Build history of the part. All positions in model axes, mm. A direction names the side the tool comes from. Give positions to 0.01 mm unless a question says otherwise; leave off trailing zeros. Loops run counter-clockwise (first coordinate to the right, second up) from the corner with the lowest first, then second, coordinate; pieces in that order, holes last. Notation, with made-up numbers: (47, 47) - (69, 47) arc R37 cw to (69, 85) - close; hole circle Ø2 at (42.5, 74.25). An arc over 180 degrees is marked (long way). Return JSON: item names as keys, results as strings. Group by question number.
1) Slice it at B-B (x = -29.4). List the corners of the cut face in (y, z).
2) Drill centre lines: probe 1 along Y at (x, z) = (-38.4, 1.1); probe 2 along Y at (x, z) = (-29.4, 1.3); probe 3 along Y at (x, z) = (-27.5, 4.05). Where is each one in solid material? Low to high. Write a range as from..to.
3) Drop flat-ended pins along their axis: pin 1 (0.6 mm diameter, centred on x = -28.5, z = 3, fed in from -Y); pin 2 (1.8 mm diameter, centred on x = -38.4, y = -23, fed in from -Z); pin 3 (1.6 mm diameter, centred on y = -2, z = 3.5, fed in from -X); pin 4 (2.5 mm diameter, centred on x = -29.4, y = 1.2, fed in from +Z). Give the stop position or say it passes through.
4) Mould opens along X. For faces 1 (the face through (-39.55, -0.35, 1.28)), 2 (the face through (-29, -3.6, 4)), 3 (the face through (-40.5, -14, 1)) say: released by +X, released by -X, zero draft, split by the parting line, or undercut.
5) Slice it at D-D (x = -38.4). List the corners of the cut face in (y, z).
6) Slice it at A-A (y = -30.2). List the corners of the cut face in (x, z).
7) 3-axis set-ups, long thin cutter, end or side, ignore diameter. For faces 4 (the face through (-30, -4, 1)), 5 (the face through (-29, -27.8, 4)), 6 (the face through (-32, -2, 4)), 7 (the face through (-29, -25, 4)), 8 (the face through (-26.3, -26, 4)): which of +Z, -Z, +X, -X, +Y, -Y reach the whole face in a straight line?
8) Slice it at C-C (z = 3.15). List the corners of the cut face in (x, y).
```python
from build123d import *

# Parameters (mm, degrees)
TYPE_C_PROFILE_R  = 1.15
TYPE_C_DEPTH      = 2.6
EXTRUDE_START     = 2.6
PROFILE_W         = 5.7
PROFILE_H         = 2.8
PROFILE_H_2       = 2.4
EXTRUDE_309_DEPTH = 2


with BuildPart() as part:
    # 接口端底座，Type-C区开口 profile → 接口端底座，Type-C区开口 (new body)
    with BuildSketch(Plane.XY):
        Polygon((-40.5, -32), (-25.2, -32), (-25.2, -14), (-35, -14), (-35, -4), (-25.2, -4), (-25.2, 3.15), (-40.5, 3.15), align=None)
        with Locations((-38.4, -23)):
            Circle(TYPE_C_PROFILE_R, mode=Mode.SUBTRACT)
        with Locations((-38.4, -0.4)):
            Circle(TYPE_C_PROFILE_R, mode=Mode.SUBTRACT)
        with Locations((-29.4, -30.2)):
            Circle(TYPE_C_PROFILE_R, mode=Mode.SUBTRACT)
        with Locations((-29.4, 1.2)):
            Circle(TYPE_C_PROFILE_R, mode=Mode.SUBTRACT)
    extrude(amount=TYPE_C_DEPTH)

    # profile → Extrude 309 (add)
    with BuildSketch(Plane.XY.offset(EXTRUDE_START)):
        with Locations((-29.15, -26.4)):
            Rectangle(PROFILE_W, PROFILE_H)
        with Locations((-29.15, -2.4)):
            Rectangle(PROFILE_W, PROFILE_H_2)
    extrude(amount=EXTRUDE_309_DEPTH)


solid = part.part
```
Results:
{
 "1": {"outline": "(-32, 0) - (-31.35, 0) - (-31.35, 2.6) - (-32, 2.6) - close; (-29.05, 0) - (-14, 0) - (-14, 2.6) - (-25, 2.6) - (-25, 4.6) - (-27.8, 4.6) - (-27.8, 2.6) - (-29.05, 2.6) - close; (-4, 0) - (0.05, 0) - (0.05, 2.6) - (-1.2, 2.6) - (-1.2, 4.6) - (-3.6, 4.6) - (-3.6, 2.6) - (-4, 2.6) - close; (2.35, 0) - (3.15, 0) - (3.15, 2.6) - (2.35, 2.6) - close"},
 "2": {"probe 1": "-32..-24.15, -21.85..-1.55, 0.75..3.15", "probe 2": "-32..-31.35, -29.05..-14, -4..0.05, 2.35..3.15", "probe 3": "-27.8..-25, -3.6..-1.2"},
 "3": {"pin 1": "y = -27.8", "pin 2": "through", "pin 3": "x = -32", "pin 4": "z = 2.6"},
 "4": {"face 1": "undercut", "face 2": "zero draft", "face 3": "released by -X"},
 "5": {"outline": "(-32, 0) - (-24.15, 0) - (-24.15, 2.6) - (-32, 2.6) - close; (-21.85, 0) - (-1.55, 0) - (-1.55, 2.6) - (-21.85, 2.6) - close; (0.75, 0) - (3.15, 0) - (3.15, 2.6) - (0.75, 2.6) - close"},
 "6": {"outline": "(-40.5, 0) - (-30.55, 0) - (-30.55, 2.6) - (-40.5, 2.6) - close; (-28.25, 0) - (-25.2, 0) - (-25.2, 2.6) - (-28.25, 2.6) - close"},
 "7": {"face 4": "+Z, -Z, +X", "face 5": "+Z, +X, -X, -Y", "face 6": "+Z, -X, +Y, -Y", "face 7": "+Z, +X, -X", "face 8": "+Z, +X, +Y, -Y"},
 "8": {"outline": "(-32, -27.8) - (-26.3, -27.8) - (-26.3, -25) - (-32, -25) - close; (-32, -3.6) - (-26.3, -3.6) - (-26.3, -1.2) - (-32, -1.2) - close"}
}
